from build123d import *

# Parameters (mm, degrees)
BOSS_EXTRUDE1_DEPTH = 100
SKETCH3_W           = 7.7
SKETCH3_H           = 7.5
CUT_EXTRUDE1_DEPTH  = 207.039437972


with BuildPart() as part:
    # Sketch1 → Boss-Extrude1 (new, symmetric)
    with BuildSketch(Plane(origin=(0, 0, 0), x_dir=(0, 0, -1), z_dir=(1, 0, 0))):
        Polygon((-48.5, 0), (48.5, 10), (48.5, 0), align=None)
    extrude(amount=BOSS_EXTRUDE1_DEPTH, both=True)

    # Sketch3 → Cut-Extrude1 (cut, through all)
    with BuildSketch(Plane(origin=(100, 0, 0), x_dir=(0, 0, -1), z_dir=(1, 0, 0))):
        with Locations((44.65, 3.75)):
            Rectangle(SKETCH3_W, SKETCH3_H)
    extrude(amount=-CUT_EXTRUDE1_DEPTH, mode=Mode.SUBTRACT)


solid = part.part
Model file for the job. Use its own axes, mm. A direction names the side the tool comes from. Coordinates: 2 decimals unless noted, no trailing zeros. Order: outer loops, then holes, each group sorted by start corner. A loop starts at its lowest first (then second) coordinate and runs counter-clockwise, first axis right, second up. Notation, with made-up numbers: M 66.25,10 L 93.25,10 A14 cw 93.25,14 Z; hole C 80,-25.5 d10. An arc over 180 degrees is marked long. Return JSON: item names as keys, results as strings.
1. Flat gauge pins, fed straight in: pin 1 (6 mm diameter, centred on x = 49, y = 4, fed in from -Z); pin 2 (3 mm diameter, centred on x = 72.5, z = 30, fed in from +Y). Where does each tip first touch, or does it go through?
Ans:
{"pin 1": "z = -40.8", "pin 2": "y = 2.06"}
2. Saw through at C-C (z = 32.5). Give the cut face in (x, y).
Ans:
{"outline": "M -100,0 L 100,0 L 100,1.65 L -100,1.65 Z"}
3. Tool access for faces 1 (the face through (-100, 4, -15)), 2 (the face through (1, 7.5, -45)): list every direction of +Z, -Z, +X, -X, +Y, -Y with a clear straight run to the whole face (end or side of a thin tool).
Ans:
{"face 1": "+Z, -Z, -X, +Y, -Y", "face 2": "-Z, +X, -X, -Y"}
4. Saw through at B-B (y = 2.5). Give the cut face in (x, z).
Ans:
{"outline": "M -100,-40.8 L 100,-40.8 L 100,24.25 L -100,24.25 Z"}
5. Drill centre lines: probe 1 along Y at (x, z) = (-3.5, -38.5); probe 2 along Y at (x, z) = (-16, -21.5). Where is each one in solid material? Low to high.
Ans:
{"probe 1": "0 to 8.97", "probe 2": "0 to 7.22"}
6. Saw through at A-A (x = -57.5). Give the cut face in (y, z).
Ans:
{"outline": "M 0,-40.8 L 7.5,-40.8 L 7.5,-48.5 L 10,-48.5 L 0,48.5 Z"}
